from build123d import *

# Parameters (mm, degrees)
F1_DEPTH = 483.87
F3_DEPTH = 76.2
F4_R     = 38.1
F5_DEPTH = 50.8
F2_R     = 63.5
F6_DEPTH = 50.8


with BuildPart() as f1:
    # F0 (on Front) → F1 (new body)
    with BuildSketch(Plane.XZ):
        with BuildLine():
            Line((323.430955, 639.79906), (-125.581851, 190.786254))
            ThreePointArc((-125.581851, 190.786254), (-149.808374, 68.9913), (-46.555597, 0))
            Line((-46.555597, 0), (1223.444403, 0))
            Line((1223.444403, 0), (1223.444403, 48.26))
            Line((1223.444403, 48.26), (-46.555597, 48.26))
            ThreePointArc((-46.555597, 48.26), (-105.221948, 87.459602), (-91.456878, 156.661281))
            Line((-91.456878, 156.661281), (357.555928, 605.674087))
            Line((357.555928, 605.674087), (323.430955, 639.79906))
        make_face()
    extrude(amount=-F1_DEPTH)

    # F2 (on face) → F3 (cut)
    with BuildSketch(Plane.XY.offset(48.26)):
        with BuildLine():
            Line((791.644403, 178.435), (1045.644403, 178.435))
            ThreePointArc((1045.644403, 178.435), (1109.144403, 241.935), (1045.644403, 305.435))
            Line((1045.644403, 305.435), (791.644403, 305.435))
            ThreePointArc((791.644403, 305.435), (728.144403, 241.935), (791.644403, 178.435))
        make_face()
    extrude(amount=-F3_DEPTH, mode=Mode.SUBTRACT)

    # F4 (on face) → F5 (cut)
    with BuildSketch(Plane(origin=(-158.184053, 0, 158.184053), x_dir=(0, -1, 0), z_dir=(-0.707107, 0, 0.707107))):
        with Locations((-369.57, 490.606475)):
            Circle(F4_R)
        with Locations((-114.3, 490.606475)):
            Circle(F4_R)
    extrude(amount=-F5_DEPTH, mode=Mode.SUBTRACT)

    # F2 (on face) → F6 (cut)
    with BuildSketch(Plane.XY.offset(48.26)):
        with Locations((410.644403, 241.935)):
            Circle(F2_R)
    extrude(amount=-F6_DEPTH, mode=Mode.SUBTRACT)


solid = f1.part
Design review of the part built by this model. Coordinates are the model's own, in mm. A direction names the side the tool comes from. Coordinates: 2 decimals unless noted, no trailing zeros. Order: outer loops, then holes, each group sorted by start corner. A loop starts at its lowest first (then second) coordinate and runs counter-clockwise, first axis right, second up.
Item 1: For line 1 (Z direction, x = 128, y = 325); line 2 (Z direction, x = 969, y = 428); line 3 (Z direction, x = 329.5, y = 237), list the stretches that pass through material, from the lowest coordinate up.
Item 2: Take a section at B-B, the plane y = 446. Write out the cut boundary in (x, z).
Item 3: Take a section at D-D, the plane x = 674. Write out the cut boundary in (y, z).
Item 4: The part is to be moulded in two halves that separate along Z. For faces 1 (the flat face through (129.906, 238.548, 378.025)), 2 (the cylindrical face through (-150.5, 238.5, 70.7)), 3 (the flat face through (102.07, 238.55, 418.44)), say which applies: pulls with the +Z half, pulls with the -Z half, needs draft (parallel to the pull), parting line crosses it, or undercut.
Item 5: For pin 1 Ø3 at (x, y) = (289.5, 305.5) entering from -Z; pin 2 Ø8 at (x, y) = (876.5, 435.5) entering from +Z; pin 3 Ø3 at (y, z) = (383, 291.5) entering from -X; pin 4 Ø6 at (y, z) = (331, 75) entering from +X, all flat-tipped, find the tip position at first contact; note any pin that passes through.
Item 6: For faces 4 (the flat face through (597, 239, 48.26)), 5 (the flat face through (340.73, 238.55, 622.5)), 6 (the cylindrical face through (728.16, 243.33, 24.47)), list the 3-axis set-ups (+Z, -Z, +X, -X, +Y, -Y) from which the entire face can be reached by the end or side of a thin tool; tool diameter is ignored.
Item 7: Take a section at C-C, the plane y = 383.5. Write out the cut boundary in (x, z).
Item 8: Take a section at A-A, the plane x = 876. Write out the cut boundary in (y, z) (3 decimals), then the cut area to 3 significant figures.
The answers:
1. line 1: z = 0 to 48.26, 376.12 to 444.37
1. line 2: z = 0 to 48.26
1. line 3: z = 0 to 48.26, 577.62 to 633.73
2. outline: (-125.58, 190.79) arc R111.76 ccw to (-46.56, 0) - (1223.44, 0) - (1223.44, 48.26) - (-46.56, 48.26) arc R63.5 cw to (-91.46, 156.66) - (357.56, 605.67) - (323.43, 639.8) - close
3. outline: (0, 0) - (483.87, 0) - (483.87, 48.26) - (0, 48.26) - close
4. face 1: undercut
4. face 2: parting line crosses it
4. face 3: pulls with the +Z half
5. pin 1: stops at z = 0
5. pin 2: stops at z = 48.26
5. pin 3: stops at x = -26.37
5. pin 4: stops at x = -96.07
6. face 4: +X, +Y, -Y
6. face 5: +Z, +X, +Y, -Y
6. face 6: +Z, -Z
7. outline: (-125.58, 190.79) arc R111.76 ccw to (-46.56, 0) - (1223.44, 0) - (1223.44, 48.26) - (-46.56, 48.26) arc R63.5 cw to (-91.46, 156.66) - (197.78, 445.89) - (163.65, 480.02) - close; (213.8, 530.17) - (247.93, 496.05) - (357.56, 605.67) - (323.43, 639.8) - close
8. outline: (0, 0) - (178.435, 0) - (178.435, 48.26) - (0, 48.26) - close; (305.435, 0) - (483.87, 0) - (483.87, 48.26) - (305.435, 48.26) - close
8. area: 17,200 mm2
